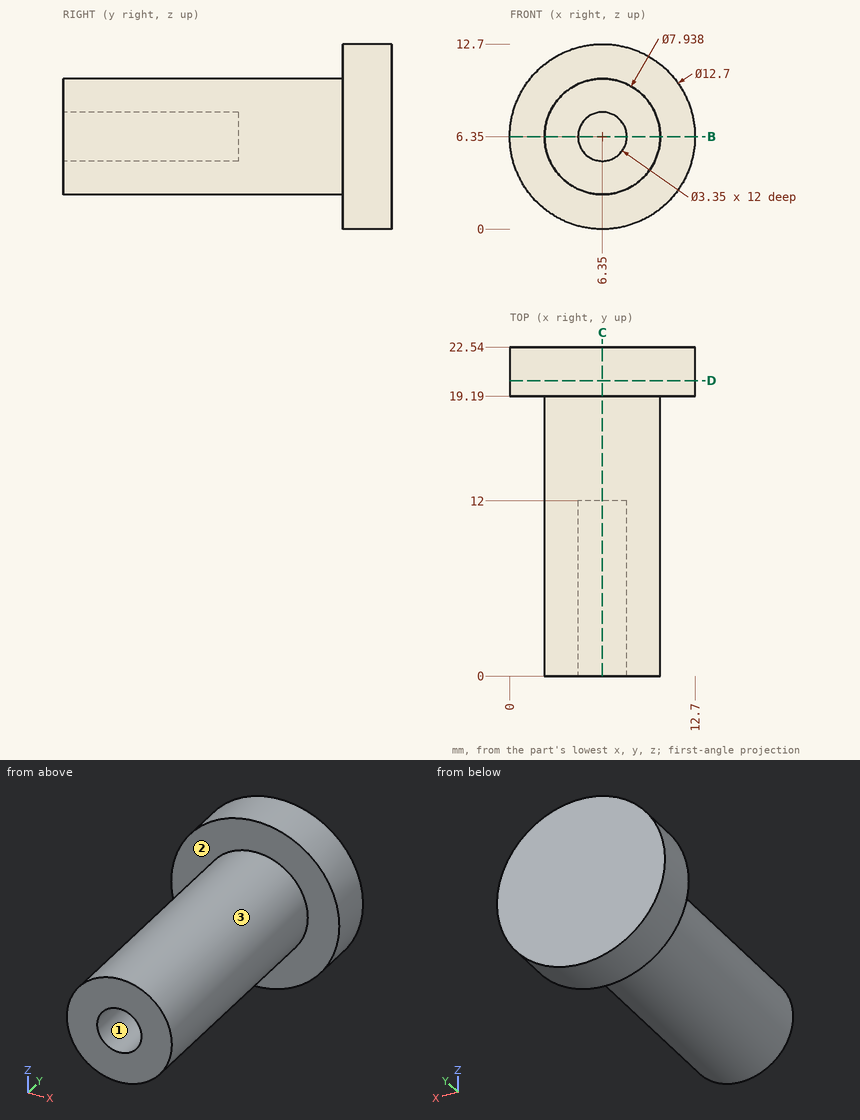
Part print with two shaded views. Sizes in mm from the minimum x, y, z corner. Give positions to 0.01 mm unless a question says otherwise; leave off trailing zeros. Loops run counter-clockwise (first coordinate to the right, second up) from the corner with the lowest first, then second, coordinate; pieces in that order, holes last. Notation, with made-up numbers: (-14, -26.75) - (27, -26.75) arc R16 ccw to (27, -20.75) - close; hole circle Ø9 at (70, 39). An arc over 180 degrees is marked (long way). Put each result on its own line as item: value.
Q1. Slice it at D-D (y = 20.25). Give the cut face in (x, z), plus the area to 3 significant figures.
Filled in:
outline: circle Ø12.7 at (6.35, 6.35)
area: 127 mm²
Q2. Probe line 1 along Z through (x, y) = (6.35, 7.5) (1 decimal); line 2 along Y through (x, z) = (1.75, 4.75); line 3 along Y through (x, z) = (6, 7.5). List the from-to ranges inside material, lowest first.
Filled in:
line 1: z = 2.4 to 4.7, 8 to 10.3
line 2: y = 19.19 to 22.54
line 3: y = 12 to 22.54
Q3. Flat gauge pins, fed straight in: pin 1 (6 mm diameter, centred on y = 12.5, z = 11, fed in from +X); pin 2 (1.5 mm diameter, centred on y = 16.5, z = 9.5, fed in from +X); pin 3 (6 mm diameter, centred on y = 9.5, z = 3.5, fed in from -X). Where does each tip first touch, or does it go through?
Filled in:
pin 1: stops at x = 9.96
pin 2: stops at x = 9.51
pin 3: stops at x = 2.38
Q4. Slice it at B-B (z = 6.35). Give the cut face in (x, y) (1 decimal), plus the area to 3 significant figures.
Filled in:
outline: (0, 19.2) - (2.4, 19.2) - (2.4, 0) - (4.7, 0) - (4.7, 12) - (8, 12) - (8, 0) - (10.3, 0) - (10.3, 19.2) - (12.7, 19.2) - (12.7, 22.5) - (0, 22.5) - close
area: 155 mm²
Q5. Slice it at C-C (x = 6.35). Give the cut face in (y, z) (1 decimal), plus the area to 3 significant figures.
Filled in:
outline: (0, 2.4) - (19.2, 2.4) - (19.2, 0) - (22.5, 0) - (22.5, 12.7) - (19.2, 12.7) - (19.2, 10.3) - (0, 10.3) - (0, 8) - (12, 8) - (12, 4.7) - (0, 4.7) - close
area: 155 mm²
Q6. Mould opens along X. For the marked faces 1, 2 and 3 say: pulls with the +X half, pulls with the -X half, needs draft (parallel to the pull), parting line crosses it, or undercut.
Filled in:
face 1: undercut
face 2: needs draft
face 3: parting line crosses it
